```python
from build123d import *

# Parameters (mm, degrees)
EXTRUDE_1_DEPTH     = 10
SKETCH_2_R          = 1.4
CUT_EXTRUDE_1_DEPTH = 72.282887147
SKETCH_4_W          = 22
SKETCH_4_H          = 7
CUT_EXTRUDE_4_DEPTH = 10
CHAMFER_2_SIZE      = 0.5
SKETCH_5_W          = 10
SKETCH_5_H          = 55
CUT_EXTRUDE_5_DEPTH = 40
EXTRUDE_2_DEPTH     = 10
FILLET_1_R          = 10
SKETCH_7_R          = 5
CUT_EXTRUDE_6_DEPTH = 6
SKETCH_8_R          = 3.1
CUT_EXTRUDE_7_DEPTH = 6
SKETCH_9_W          = 40
SKETCH_9_H          = 45
CUT_EXTRUDE_8_DEPTH = 63.299678972
FILLET_2_R          = 10
FILLET_3_R          = 5
CHAMFER_3_SIZE      = 2


# Some blends are built 0.0001 mm under size
with BuildPart() as part:
    # 草图1 → 凸台-拉伸1 (new body)
    with BuildSketch(Plane(origin=(0, 0, 0), x_dir=(0, 0, -1), z_dir=(1, 0, 0))):
        with BuildLine():
            Line((-27.5, 0), (-27.5, -65))
            Line((-27.5, -65), (27.5, -65))
            Line((27.5, -65), (27.5, 0))
            ThreePointArc((27.5, 0), (0, 27.5), (-27.5, 0))
        make_face()
    extrude(amount=EXTRUDE_1_DEPTH)

    # 草图2 → 切除-拉伸1 (cut, through all)
    with BuildSketch(Plane(origin=(10, 0, 0), x_dir=(0, 0, -1), z_dir=(1, 0, 0))):
        with Locations((-9, 5.5)):
            Circle(SKETCH_2_R)
        with Locations((9, 5.5)):
            Circle(SKETCH_2_R)
        with Locations((9, -5.5)):
            Circle(SKETCH_2_R)
        with Locations((-9, -5.5)):
            Circle(SKETCH_2_R)
    extrude(amount=-CUT_EXTRUDE_1_DEPTH, mode=Mode.SUBTRACT)

    # 草图4 → 切除-拉伸4 (cut)
    with BuildSketch(Plane.ZY):
        with Locations((0, 16.5)):
            Rectangle(SKETCH_4_W, SKETCH_4_H)
    extrude(amount=-CUT_EXTRUDE_4_DEPTH, mode=Mode.SUBTRACT)

    # 倒角2
    chamfer_2_edges = [part.edges().sort_by_distance(p)[0] for p in [
        (10, 16.5, -11),
        (10, 20, 0),
        (10, 16.5, 11),
        (10, 13, 0),
        (0, 16.5, -11),
        (0, 13, 0),
        (0, 16.5, 11),
        (0, 20, 0),
    ]]
    chamfer(chamfer_2_edges, length=CHAMFER_2_SIZE)

    # 草图5 → 切除-拉伸5 (cut)
    with BuildSketch(Plane(origin=(0, -65, 0), x_dir=(-1, 0, 0), z_dir=(0, -1, 0))):
        with Locations((-5, 0)):
            Rectangle(SKETCH_5_W, SKETCH_5_H)
    extrude(amount=-CUT_EXTRUDE_5_DEPTH, mode=Mode.SUBTRACT)

    # 草图6 → 凸台-拉伸2 (add)
    with BuildSketch(Plane(origin=(0, -25, 0), x_dir=(-1, 0, 0), z_dir=(0, -1, 0))):
        Polygon((0, -27.5), (0, 27.5), (0, 47.5), (-20, 47.5), (-20, 27.5), (-20, -27.5), (-20, -47.5), (0, -47.5), align=None)
    extrude(amount=EXTRUDE_2_DEPTH)

    # 圆角1
    fillet_1_edges = [part.edges().sort_by_distance(p)[0] for p in [
        (0, -30, -47.5),
        (20, -30, -47.5),
        (0, -30, 47.5),
        (20, -30, 47.5),
    ]]
    fillet(fillet_1_edges, radius=FILLET_1_R - 0.0001)  # a hair under: the kernel refuses the full size

    # 草图7 → 切除-拉伸6 (cut)
    with BuildSketch(Plane(origin=(0, -25, 0), x_dir=(1, 0, 0), z_dir=(0, 1, 0))):
        with Locations(Location((10, 37.5, 0), (0, 0, 270))):
            Circle(SKETCH_7_R)
        with Locations(Location((10, -37.5, 0), (0, 0, 270))):
            Circle(SKETCH_7_R)
    extrude(amount=-CUT_EXTRUDE_6_DEPTH, mode=Mode.SUBTRACT)

    # 草图8 → 切除-拉伸7 (cut)
    with BuildSketch(Plane(origin=(0, -31, 0), x_dir=(1, 0, 0), z_dir=(0, 1, 0))):
        with Locations(Location((10, 37.5, 0), (0, 0, 270))):
            Circle(SKETCH_8_R)
        with Locations(Location((10, -37.5, 0), (0, 0, 270))):
            Circle(SKETCH_8_R)
    extrude(amount=-CUT_EXTRUDE_7_DEPTH, mode=Mode.SUBTRACT)

    # 草图9 → 切除-拉伸8 (cut, through all)
    with BuildSketch(Plane.ZY):
        with Locations((0, -35)):
            Rectangle(SKETCH_9_W, SKETCH_9_H)
    extrude(amount=-CUT_EXTRUDE_8_DEPTH, mode=Mode.SUBTRACT)

    # 圆角2
    fillet_2_edges = [part.edges().sort_by_distance(p)[0] for p in [
        (5, -12.5, 20),
        (5, -12.5, -20),
    ]]
    fillet(fillet_2_edges, radius=FILLET_2_R)

    # 圆角3
    fillet_3_edges = [part.edges().sort_by_distance(p)[0] for p in [
        (10, -25, -23.75),
        (10, -25, 23.75),
    ]]
    fillet(fillet_3_edges, radius=FILLET_3_R)

    # 倒角3
    # the kernel refuses this chamfer: 2 mm, written as the material it takes off along each edge
    with BuildSketch(Plane(origin=(0, -25, 37.5001), x_dir=(1, 0, 0), z_dir=(0, 0, -1)), Plane(origin=(0, -25, -27.5), x_dir=(1, 0, 0), z_dir=(0, 0, -1))) as chamfer_3_piece_1:
        Polygon((CHAMFER_3_SIZE, 0), (0, CHAMFER_3_SIZE), (0, 0), align=None)
    extrude(amount=10.0001, mode=Mode.SUBTRACT)
    with BuildSketch(Plane(origin=(20, -25, -37.5001), x_dir=(0, -1, 0), z_dir=(0, 0, 1))) as chamfer_3_piece_2:
        Polygon((CHAMFER_3_SIZE, 0), (0, -CHAMFER_3_SIZE), (0, 0), align=None)
    extrude(amount=22.643465976, mode=Mode.SUBTRACT)
    with BuildSketch(Plane(origin=(10.0001, -25, 37.5001), x_dir=(0, 0, 1), z_dir=(-1, 0, 0))) as chamfer_3_piece_3:
        Polygon((9.9999 - CHAMFER_3_SIZE, 0), (9.9999, -CHAMFER_3_SIZE), (9.9999, 0), align=None)
    revolve(axis=Axis((10.0001, -25, 37.5001), (0, 1, 0)), revolution_arc=90, mode=Mode.SUBTRACT)
    with BuildSketch(Plane(origin=(9.9999, -25, 37.5001), x_dir=(-1, 0, 0), z_dir=(0, 0, -1))) as chamfer_3_piece_4:
        Polygon((9.9999 - CHAMFER_3_SIZE, 0), (9.9999, -CHAMFER_3_SIZE), (9.9999, 0), align=None)
    revolve(axis=Axis((9.9999, -25, 37.5001), (0, 1, 0)), revolution_arc=90, mode=Mode.SUBTRACT)
    with BuildSketch(Plane(origin=(10.0001, -25, -37.5001), x_dir=(0, 0, -1), z_dir=(-1, 0, 0))) as chamfer_3_piece_5:
        Polygon((9.9999, CHAMFER_3_SIZE), (9.9999 - CHAMFER_3_SIZE, 0), (9.9999, 0), align=None)
    revolve(axis=Axis((10.0001, -25, -37.5001), (0, -1, 0)), revolution_arc=90, mode=Mode.SUBTRACT)
    with BuildSketch(Plane(origin=(9.9999, -25, -37.5001), x_dir=(-1, 0, 0), z_dir=(0, 0, 1))) as chamfer_3_piece_6:
        Polygon((9.9999, CHAMFER_3_SIZE), (9.9999 - CHAMFER_3_SIZE, 0), (9.9999, 0), align=None)
    revolve(axis=Axis((9.9999, -25, -37.5001), (0, -1, 0)), revolution_arc=90, mode=Mode.SUBTRACT)
    with BuildSketch(Plane(origin=(20, -25, 14.856634024), x_dir=(-1, 0, 0), z_dir=(0, 0, 1))) as chamfer_3_piece_7:
        Polygon((CHAMFER_3_SIZE, 0), (0, CHAMFER_3_SIZE), (0, 0), align=None)
    extrude(amount=22.643465976, mode=Mode.SUBTRACT)
    with BuildSketch(Plane(origin=(0, -40.143365976, 20), x_dir=(1, 0, 0), z_dir=(0, 1, 0)), Plane(origin=(0, -22.5, -20), x_dir=(1, 0, 0), z_dir=(0, -1, 0))) as chamfer_3_piece_8:
        Polygon((CHAMFER_3_SIZE, 0), (0, -CHAMFER_3_SIZE), (0, 0), align=None)
    extrude(amount=17.643365976, mode=Mode.SUBTRACT)
    with BuildSketch(Plane(origin=(20, -40.143365976, 20), x_dir=(0, 0, 1), z_dir=(0, 1, 0))) as chamfer_3_piece_9:
        Polygon((CHAMFER_3_SIZE, 0), (0, -CHAMFER_3_SIZE), (0, 0), align=None)
    extrude(amount=20.286731952, mode=Mode.SUBTRACT)
    with BuildSketch(Plane(origin=(20, -19.856634024, -20), x_dir=(-1, 0, 0), z_dir=(0, -1, 0))) as chamfer_3_piece_10:
        Polygon((CHAMFER_3_SIZE, 0), (0, CHAMFER_3_SIZE), (0, 0), align=None)
    extrude(amount=20.286731952, mode=Mode.SUBTRACT)
    with BuildSketch(Plane(origin=(0, -12.5, 10), x_dir=(1, 0, 0), z_dir=(0, 0, -1))) as chamfer_3_piece_11:
        Polygon((CHAMFER_3_SIZE, 0), (0, -CHAMFER_3_SIZE), (0, 0), align=None)
    extrude(amount=20, mode=Mode.SUBTRACT)
    with BuildSketch(Plane(origin=(0, -22.5, -10), x_dir=(0, 0, -1), z_dir=(0, -1, 0))) as chamfer_3_piece_12:
        Polygon((10 + CHAMFER_3_SIZE, 0), (10, CHAMFER_3_SIZE), (10, 0), align=None)
    revolve(axis=Axis((0, -22.5, -10), (1, 0, 0)), revolution_arc=90, mode=Mode.SUBTRACT)
    with BuildSketch(Plane(origin=(0, -22.5, 10), x_dir=(0, 1, 0), z_dir=(0, 0, -1))) as chamfer_3_piece_13:
        Polygon((10, CHAMFER_3_SIZE), (10 + CHAMFER_3_SIZE, 0), (10, 0), align=None)
    revolve(axis=Axis((0, -22.5, 10), (1, 0, 0)), revolution_arc=90, mode=Mode.SUBTRACT)
    with BuildSketch(Plane(origin=(10, -20, -27.5), x_dir=(-1, 0, 0), z_dir=(0, 1, 0)), Plane(origin=(10, 0, 27.5), x_dir=(-1, 0, 0), z_dir=(0, -1, 0))) as chamfer_3_piece_14:
        Polygon((CHAMFER_3_SIZE, 0), (0, CHAMFER_3_SIZE), (0, 0), align=None)
    extrude(amount=20, mode=Mode.SUBTRACT)
    with BuildSketch(Plane(origin=(15, -20, -27.5), x_dir=(0.8568283041143762, -0.5156018398614208, 0), z_dir=(0.5156018398614208, 0.8568283041143762, 0))) as chamfer_3_piece_15_section:
        Polygon((5 + CHAMFER_3_SIZE, 0), (5, -CHAMFER_3_SIZE), (5, 0), align=None)
    chamfer_3_piece_15 = revolve(axis=Axis((15, -20, -27.5), (0, 0, -1)), revolution_arc=148.962308712, mode=Mode.PRIVATE)
    chamfer_3_piece_15 = split(chamfer_3_piece_15, bisect_by=Plane(origin=(15, -25, -27.5), z_dir=(0, 1, 0)), keep=Keep.TOP, mode=Mode.PRIVATE)
    add(chamfer_3_piece_15, mode=Mode.SUBTRACT)
    with BuildSketch(Plane(origin=(15, -20, 27.5), x_dir=(0.8568283041143756, -0.5156018398614214, 0), z_dir=(0.5156018398614214, 0.8568283041143756, 0))) as chamfer_3_piece_16_section:
        Polygon((5 + CHAMFER_3_SIZE, 0), (5, CHAMFER_3_SIZE), (5, 0), align=None)
    chamfer_3_piece_16 = revolve(axis=Axis((15, -20, 27.5), (0, 0, -1)), revolution_arc=148.962308712, mode=Mode.PRIVATE)
    chamfer_3_piece_16 = split(chamfer_3_piece_16, bisect_by=Plane(origin=(15, -25, 27.5), z_dir=(0, 1, 0)), keep=Keep.TOP, mode=Mode.PRIVATE)
    add(chamfer_3_piece_16, mode=Mode.SUBTRACT)
    with BuildSketch(Plane(origin=(10, 0, 0), x_dir=(0, 0, -1), z_dir=(0, -1, 0))) as chamfer_3_piece_17:
        Polygon((27.5, -CHAMFER_3_SIZE), (27.5 - CHAMFER_3_SIZE, 0), (27.5, 0), align=None)
    revolve(axis=Axis((10, 0, 0), (1, 0, 0)), revolution_arc=180, mode=Mode.SUBTRACT)
    with BuildSketch(Plane(origin=(0, 0, 27.5), x_dir=(1, 0, 0), z_dir=(0, -1, 0)), Plane(origin=(0, -25, -27.5), x_dir=(1, 0, 0), z_dir=(0, 1, 0))) as chamfer_3_piece_18:
        Polygon((CHAMFER_3_SIZE, 0), (0, -CHAMFER_3_SIZE), (0, 0), align=None)
    extrude(amount=25, mode=Mode.SUBTRACT)
    with BuildSketch(Plane(origin=(0, 0, 0), x_dir=(0, 0, -1), z_dir=(0, -1, 0))) as chamfer_3_piece_19:
        Polygon((27.5, CHAMFER_3_SIZE), (27.5 - CHAMFER_3_SIZE, 0), (27.5, 0), align=None)
    revolve(axis=Axis((0, 0, 0), (1, 0, 0)), revolution_arc=180, mode=Mode.SUBTRACT)
    with BuildSketch(Plane(origin=(9.9999, -25, -47.5), x_dir=(0, -1, 0), z_dir=(1, 0, 0))) as chamfer_3_piece_20:
        Polygon((CHAMFER_3_SIZE, 0), (0, -CHAMFER_3_SIZE), (0, 0), align=None)
    extrude(amount=0.0002, mode=Mode.SUBTRACT)
    with BuildSketch(Plane(origin=(10.0001, -25, 47.5), x_dir=(0, 0, -1), z_dir=(-1, 0, 0))) as chamfer_3_piece_21:
        Polygon((CHAMFER_3_SIZE, 0), (0, CHAMFER_3_SIZE), (0, 0), align=None)
    extrude(amount=0.0002, mode=Mode.SUBTRACT)
    with BuildSketch(Plane(origin=(0, 0, 27.5), x_dir=(1, 0, 0), z_dir=(0, -1, 0))) as chamfer_3_piece_22a_section:
        Polygon((CHAMFER_3_SIZE, 0), (0, -CHAMFER_3_SIZE), (0, 0), align=None)
    chamfer_3_piece_22a = extrude(amount=30.143365976, mode=Mode.PRIVATE)
    chamfer_3_piece_22a = split(chamfer_3_piece_22a, bisect_by=Plane(origin=(0, -25, 27.5), z_dir=(0, -1, 0)), keep=Keep.TOP, mode=Mode.PRIVATE)
    with BuildSketch(Plane(origin=(0, -25, 37.5001), x_dir=(1, 0, 0), z_dir=(0, 0, -1))) as chamfer_3_piece_22b_section:
        Polygon((CHAMFER_3_SIZE, 0), (0, CHAMFER_3_SIZE), (0, 0), align=None)
    chamfer_3_piece_22b = extrude(amount=15.143465976, mode=Mode.PRIVATE)
    chamfer_3_piece_22b = split(chamfer_3_piece_22b, bisect_by=Plane(origin=(0, -25, 27.5), z_dir=(0, 0, -1)), keep=Keep.TOP, mode=Mode.PRIVATE)
    chamfer_3_piece_22 = chamfer_3_piece_22a & chamfer_3_piece_22b
    add(chamfer_3_piece_22, mode=Mode.SUBTRACT)
    with BuildSketch(Plane(origin=(0, -25, -22.356634024), x_dir=(1, 0, 0), z_dir=(0, 0, -1))) as chamfer_3_piece_23a_section:
        Polygon((CHAMFER_3_SIZE, 0), (0, CHAMFER_3_SIZE), (0, 0), align=None)
    chamfer_3_piece_23a = extrude(amount=15.143465976, mode=Mode.PRIVATE)
    chamfer_3_piece_23a = split(chamfer_3_piece_23a, bisect_by=Plane(origin=(0, -25, -27.5), z_dir=(0, 0, 1)), keep=Keep.TOP, mode=Mode.PRIVATE)
    with BuildSketch(Plane(origin=(0, -30.143365976, -27.5), x_dir=(1, 0, 0), z_dir=(0, 1, 0))) as chamfer_3_piece_23b_section:
        Polygon((CHAMFER_3_SIZE, 0), (0, -CHAMFER_3_SIZE), (0, 0), align=None)
    chamfer_3_piece_23b = extrude(amount=30.143365976, mode=Mode.PRIVATE)
    chamfer_3_piece_23b = split(chamfer_3_piece_23b, bisect_by=Plane(origin=(0, -25, -27.5), z_dir=(0, -1, 0)), keep=Keep.TOP, mode=Mode.PRIVATE)
    chamfer_3_piece_23 = chamfer_3_piece_23a & chamfer_3_piece_23b
    add(chamfer_3_piece_23, mode=Mode.SUBTRACT)


solid = part.part
```
Part model, mm, in its own coordinate system. A direction names the side the tool comes from. Give positions to 0.01 mm unless a question says otherwise; leave off trailing zeros. Write each loop counter-clockwise with the first axis right and the second up, starting at its lowest first coordinate (ties: lowest second). Pieces come first, ordered by that corner, then holes. Notation, with made-up numbers: M 1.25,-30 L 34.25,-30 A31 ccw 34.25,-5 Z; hole C 7,24 d9. An arc over 180 degrees is marked long. Use CSV: the item, a comma, the result in double quotes.
Item 1: Which spindle directions (+Z, -Z, +X, -X, +Y, -Y) get a long thin tool onto all of the face, cutting with end or side? Do faces 4 (the face through (9, -9.9, 26.5)), 5 (the face through (1, -13.7, -26.5)), 6 (the face through (5, -13, 27.5)). Say none if no direction does.
Taken from the geometry:
face 4,"+Z, +X, +Y"
face 5,"-Z, -X, +Y"
face 6,"+Z, +X, -X, +Y"
Item 2: Slice it at B-B on z = -29. Write the cut outline in (x, y), plus the area to 3 significant figures.
Taken from the geometry:
outline,"M 0,-35 L 20,-35 L 20,-27 L 18,-25 L 2,-25 L 0,-27 Z"
area,"196 mm²"
Item 3: Slice it at A-A on z = 0. Write the cut outline in (x, y), plus the area to 4 significant figures.
Taken from the geometry:
outline,"M 0,-10.5 L 2,-12.5 L 10,-12.5 L 10,12.5 L 9.5,13 L 0.5,13 L 0,12.5 Z; M 0,20.5 L 0.5,20 L 9.5,20 L 10,20.5 L 10,25.5 L 8,27.5 L 2,27.5 L 0,25.5 Z"
area,"323.5 mm²"
Item 4: Drill centre lines: probe 1 along Y at (x, z) = (5.25, -9); probe 2 along Z at (x, y) = (2, -3); probe 3 along Y at (x, z) = (4.75, 4). Where is each one in solid material? Low to high.
Taken from the geometry:
probe 1,"y = -12.5 to -6.9, -4.1 to 4.1, 6.9 to 13, 20 to 25.99"
probe 2,"z = -27.5 to 27.5"
probe 3,"y = -12.5 to 13, 20 to 27.21"
Item 5: Pin check, flat tips, straight feed: P1, Ø2.5, axis at x = 4, z = -4.5, coming from the +Y side; P2, Ø9, axis at x = 10, z = -37.5, coming from the +Y side; P3, Ø2, axis at x = 4.5, y = -14, coming from the +Z side. Stop position of each tip, or through.
Taken from the geometry:
P1,"stops at y = 27.31"
P2,"stops at y = -31"
P3,"stops at z = 27.5"
Item 6: Slice it at C-C on x = 4. State how many separate pieces and enclosed holes the cut face has, plus the area to 3 significant figures.
Taken from the geometry:
separate pieces,"1"
enclosed holes,"5"
area,"2,430 mm²"
Item 7: Pull direction Y, two halves, no side cores. Call faces 1 (the face through (9.681, 25.813, -0.568)), 2 (the face through (5.07, 5.56, -7.6)), 3 (the face through (3.01, -31.06, -44.65)): +Y half, -Y half, draft (parallel to the pull), parting line (faces both ways), or undercut.
Taken from the geometry:
face 1,"+Y half"
face 2,"undercut"
face 3,"draft"
